Could you check a few things on this drawing? It's one solid part, dimensions in mm from its lowest x, y, z. Round coordinates to 2 decimals unless told otherwise and drop trailing zeros. Write each loop counter-clockwise with the first axis right and the second up, starting at its lowest first coordinate (ties: lowest second). Pieces come first, ordered by that corner, then holes. Notation, with made-up numbers: (-3.5, 81.25) - (48.5, 81.25) arc R6 ccw to (48.5, 85.25) - close; hole circle Ø3 at (5, 51.5). An arc over 180 degrees is marked (long way). Put each result on its own line as item: value.
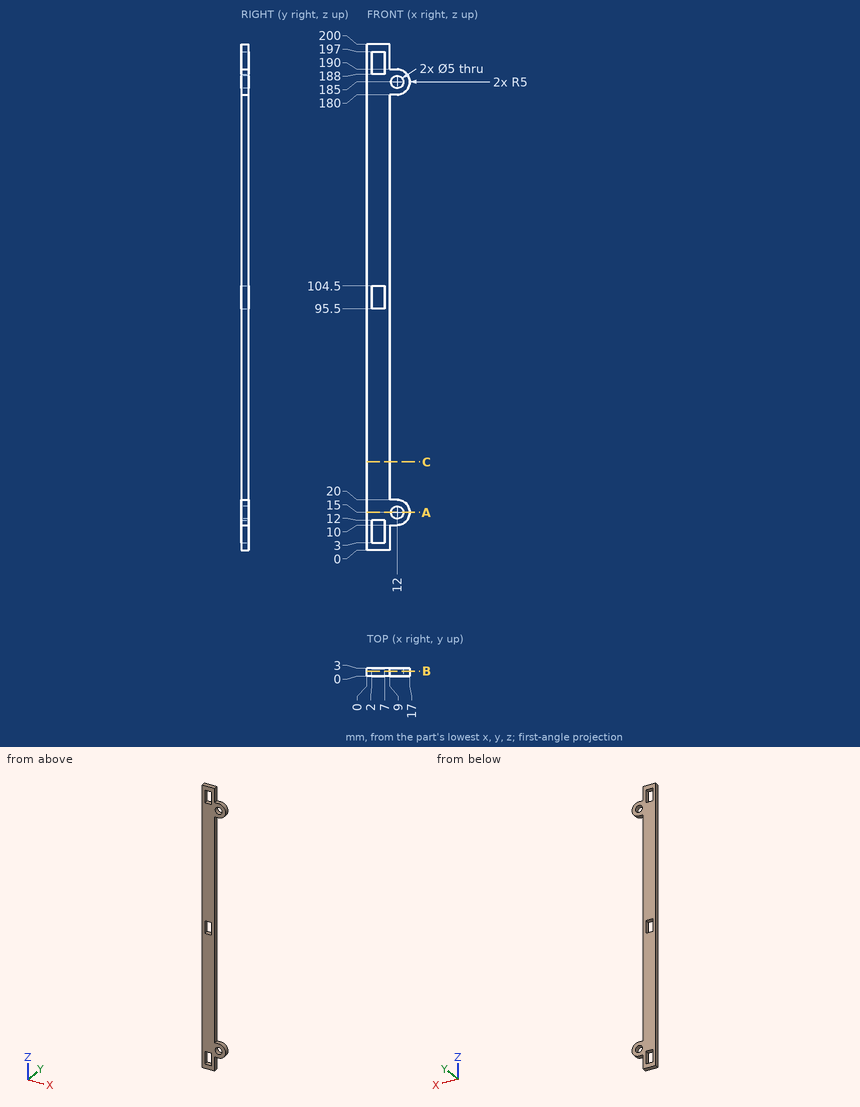
(1) Imagine slicing it at C-C, the plane z = 35. List the corners of the cut face in (x, y) for me, then the cut area to 3 significant figures.
Values found:
outline: (0, 0) - (9, 0) - (9, 3) - (0, 3) - close
area: 27.0 mm^2
(2) Please list where these lines run through material, in increasing order: probe 1 along Z at (x, y) = (6.25, 2.3); probe 2 along Z at (x, y) = (12, 1.25); probe 3 along X at (y, z) = (0.7, 185). Write a range as from..to.
Values found:
probe 1: z = 0..3, 12..95.5, 104.5..188, 197..200
probe 2: z = 10..12.5, 17.5..20, 180..182.5, 187.5..190
probe 3: x = 0..9.5, 14.5..17
(3) I'm going to push flat-ended pins straight in: pin 1 (1.5 mm diameter, centred on y = 0.5, z = 150, fed in from -X); pin 2 (1.5 mm diameter, centred on y = 1, z = 192, fed in from +X); pin 3 (1.5 mm diameter, centred on x = 10, y = 1, fed in from -Z); pin 4 (0.9 mm diameter, centred on x = 10, y = 1.5, fed in from +Z). Where does each tip first touch, or does it pass through?
Values found:
pin 1: stops at x = 0
pin 2: stops at x = 9
pin 3: stops at z = 10
pin 4: stops at z = 190
(4) Imagine slicing it at A-A, the plane z = 15. List the corners of the cut face in (x, y) for me, then the cut area to 3 significant figures.
Values found:
outline: (0, 0) - (9.5, 0) - (9.5, 3) - (0, 3) - close; (14.5, 0) - (17, 0) - (17, 3) - (14.5, 3) - close
area: 36.0 mm^2
(5) Imagine slicing it at B-B, the plane y = 1.9. List the corners of the cut face in (x, z) for me.
Values found:
outline: (0, 0) - (9, 0) - (9, 10) - (12, 10) arc R5 ccw to (12, 20) - (9, 20) - (9, 180) - (12, 180) arc R5 ccw to (12, 190) - (9, 190) - (9, 200) - (0, 200) - close; hole (2, 3) - (7, 3) - (7, 12) - (2, 12) - close; hole (2, 95.5) - (7, 95.5) - (7, 104.5) - (2, 104.5) - close; hole (2, 188) - (7, 188) - (7, 197) - (2, 197) - close; hole circle Ø5 at (12, 15); hole circle Ø5 at (12, 185)
